Check sheet for the modelled part. Datum: model origin and axes. Units: mm. Face numbers are marked on the shaded views. Give positions to 0.01 mm unless a question says otherwise; leave off trailing zeros. Order: outer loops, then holes, each group sorted by start corner. A loop starts at its lowest first (then second) coordinate and runs counter-clockwise, first axis right, second up.
```python
from build123d import *

# Parameters (mm, degrees)
F1_DEPTH = 1.2
F2_R     = 14
F2_R_2   = 13
F3_DEPTH = 9
F5_DEPTH = 25


with BuildPart() as f1:
    # F0 (on Top) → F1 (new body)
    with BuildSketch(Plane.XY):
        with BuildLine():
            ThreePointArc((0, 55), (-38.890873, 38.890873), (-55, 0))
            ThreePointArc((-55, 0), (-38.890873, -38.890873), (0, -55))
            ThreePointArc((0, -55), (38.890873, -38.890873), (55, 0))
            ThreePointArc((55, 0), (38.890873, 38.890873), (0, 55))
        make_face()
        with BuildLine():
            ThreePointArc((-6, -41.024383), (-7.11965, -43.361964), (-9.642857, -43.954696))
            ThreePointArc((-9.642857, -43.954696), (-31.819805, -31.819805), (-43.954696, -9.642857))
            ThreePointArc((-43.954696, -9.642857), (-43.361964, -7.11965), (-41.024383, -6))
            Line((-41.024383, -6), (-15.588457, -6))
            ThreePointArc((-15.588457, -6), (-14.088457, -6.401924), (-12.990381, -7.5))
            ThreePointArc((-12.990381, -7.5), (-10.606602, -10.606602), (-7.5, -12.990381))
            ThreePointArc((-7.5, -12.990381), (-6.401924, -14.088457), (-6, -15.588457))
            Line((-6, -15.588457), (-6, -41.024383))
        make_face(mode=Mode.SUBTRACT)
        with BuildLine():
            ThreePointArc((41.024383, -6), (43.361964, -7.11965), (43.954696, -9.642857))
            ThreePointArc((43.954696, -9.642857), (31.819805, -31.819805), (9.642857, -43.954696))
            ThreePointArc((9.642857, -43.954696), (7.11965, -43.361964), (6, -41.024383))
            Line((6, -41.024383), (6, -15.588457))
            ThreePointArc((6, -15.588457), (6.401924, -14.088457), (7.5, -12.990381))
            ThreePointArc((7.5, -12.990381), (10.606602, -10.606602), (12.990381, -7.5))
            ThreePointArc((12.990381, -7.5), (14.088457, -6.401924), (15.588457, -6))
            Line((15.588457, -6), (41.024383, -6))
        make_face(mode=Mode.SUBTRACT)
        with BuildLine():
            ThreePointArc((-7.5, 12.990381), (-10.606602, 10.606602), (-12.990381, 7.5))
            ThreePointArc((-12.990381, 7.5), (-14.088457, 6.401924), (-15.588457, 6))
            Line((-15.588457, 6), (-41.024383, 6))
            ThreePointArc((-41.024383, 6), (-43.361964, 7.11965), (-43.954696, 9.642857))
            ThreePointArc((-43.954696, 9.642857), (-31.819805, 31.819805), (-9.642857, 43.954696))
            ThreePointArc((-9.642857, 43.954696), (-7.11965, 43.361964), (-6, 41.024383))
            Line((-6, 41.024383), (-6, 15.588457))
            ThreePointArc((-6, 15.588457), (-6.401924, 14.088457), (-7.5, 12.990381))
        make_face(mode=Mode.SUBTRACT)
        with BuildLine():
            ThreePointArc((6, 41.024383), (7.11965, 43.361964), (9.642857, 43.954696))
            ThreePointArc((9.642857, 43.954696), (31.819805, 31.819805), (43.954696, 9.642857))
            ThreePointArc((43.954696, 9.642857), (43.361964, 7.11965), (41.024383, 6))
            Line((41.024383, 6), (15.588457, 6))
            ThreePointArc((15.588457, 6), (14.088457, 6.401924), (12.990381, 7.5))
            ThreePointArc((12.990381, 7.5), (10.606602, 10.606602), (7.5, 12.990381))
            ThreePointArc((7.5, 12.990381), (6.401924, 14.088457), (6, 15.588457))
            Line((6, 15.588457), (6, 41.024383))
        make_face(mode=Mode.SUBTRACT)
    extrude(amount=F1_DEPTH)

    # F2 (on Top) → F3 (join)
    with BuildSketch(Plane.XY):
        Circle(F2_R)
        Circle(F2_R_2, mode=Mode.SUBTRACT)
    extrude(amount=F3_DEPTH)

    # F4 (on Top) → F5 (cut)
    with BuildSketch(Plane.XY):
        with BuildLine():
            ThreePointArc((-6.149095, -2.106806), (-5.916805, -2.690989), (-5.629165, -3.25))
            ThreePointArc((-5.629165, -3.25), (-5.288867, -3.778608), (-4.899095, -4.271869))
            ThreePointArc((-4.899095, -4.271869), (0, -6.5), (4.899095, -4.271869))
            ThreePointArc((4.899095, -4.271869), (5.288867, -3.778608), (5.629165, -3.25))
            ThreePointArc((5.629165, -3.25), (5.916805, -2.690989), (6.149095, -2.106806))
            ThreePointArc((6.149095, -2.106806), (5.629165, 3.25), (1.25, 6.378675))
            ThreePointArc((1.25, 6.378675), (0.627937, 6.469598), (0, 6.5))
            ThreePointArc((0, 6.5), (-0.627937, 6.469598), (-1.25, 6.378675))
            ThreePointArc((-1.25, 6.378675), (-5.629165, 3.25), (-6.149095, -2.106806))
        make_face()
        with BuildLine():
            ThreePointArc((-4.899095, -4.271869), (-5.288867, -3.778608), (-5.629165, -3.25))
            ThreePointArc((-5.629165, -3.25), (-5.916805, -2.690989), (-6.149095, -2.106806))
            Line((-6.149095, -2.106806), (-8.592399, -3.517448))
            ThreePointArc((-8.592399, -3.517448), (-9.211654, -4.277101), (-9.093267, -5.25))
            ThreePointArc((-9.093267, -5.25), (-8.309905, -5.838976), (-7.342399, -5.682512))
            Line((-7.342399, -5.682512), (-4.899095, -4.271869))
        make_face()
        with BuildLine():
            ThreePointArc((5.629165, -3.25), (5.288867, -3.778608), (4.899095, -4.271869))
            Line((4.899095, -4.271869), (7.342399, -5.682512))
            ThreePointArc((7.342399, -5.682512), (8.309905, -5.838976), (9.093267, -5.25))
            ThreePointArc((9.093267, -5.25), (9.211654, -4.277101), (8.592399, -3.517448))
            Line((8.592399, -3.517448), (6.149095, -2.106806))
            ThreePointArc((6.149095, -2.106806), (5.916805, -2.690989), (5.629165, -3.25))
        make_face()
        with BuildLine():
            Line((-1.25, 9.19996), (-1.25, 6.378675))
            ThreePointArc((-1.25, 6.378675), (-0.627937, 6.469598), (0, 6.5))
            ThreePointArc((0, 6.5), (0.627937, 6.469598), (1.25, 6.378675))
            Line((1.25, 6.378675), (1.25, 9.19996))
            ThreePointArc((1.25, 9.19996), (0.901749, 10.116077), (0, 10.5))
            ThreePointArc((0, 10.5), (-0.901749, 10.116077), (-1.25, 9.19996))
        make_face()
    extrude(amount=F5_DEPTH, mode=Mode.SUBTRACT)


solid = f1.part
```
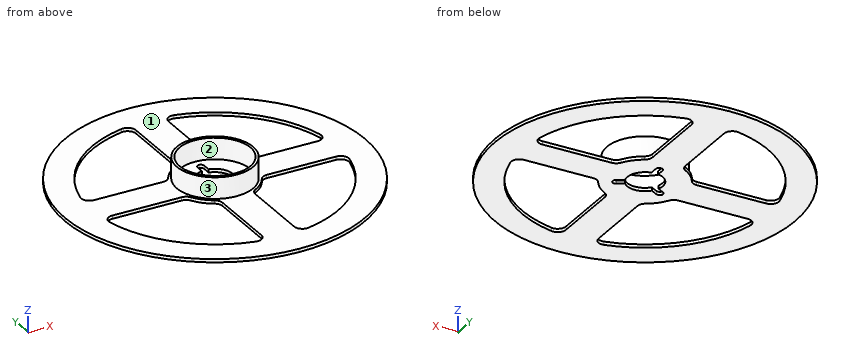
(1) Thickness scan on L1, parallel to Y at x = 0, z = 4.25; L2, parallel to X at y = -41, z = 0.5. Record the ranges inside material, lowest first.
(2) Release check for a two-part mould opening along X. For the marked faces 1, 2 and 3 record: released by +X, released by -X, zero draft, split by the parting line, or undercut.
(3) Sectioned sample at C-C (x = 3). Enter the section's corners in (y, z).
(4) Sectioned sample at B-B (y = -34). Enter the section's corners in (x, z).
(5) Go/stop test with flat-tipped pins: P1, Ø2, axis at y = -1, z = 5.5, coming from the +X side; P2, Ø1, axis at x = -40.5, y = 20, coming from the +Z side; P3, Ø0.6, axis at y = 22, z = 0.5, coming from the +X side; P4, Ø8, axis at x = -14, y = 14.5, coming from the -Z side. Record where each tip stops, or that it passes through.
(6) Sectioned sample at A-A (x = 17). Enter the section's corners in (y, z), plus the area to 3 significant figures.
(7) Sectioned sample at D-D (z = 3.25). Enter the section's corners in (x, y).
Values follow:
1. L1: y = -14 to -13, 13 to 14
1. L2: x = -36.66 to -18.55, -6 to 6, 18.55 to 36.66
2. face 1: zero draft
2. face 2: undercut
2. face 3: split by the parting line
3. outline: (-54.92, 0) - (-5.77, 0) - (-5.77, 1.2) - (-12.65, 1.2) - (-12.65, 9) - (-13.67, 9) - (-13.67, 1.2) - (-54.92, 1.2) - close; (5.77, 0) - (54.92, 0) - (54.92, 1.2) - (13.67, 1.2) - (13.67, 9) - (12.65, 9) - (12.65, 1.2) - (5.77, 1.2) - close
4. outline: (-43.23, 0) - (-29.48, 0) - (-29.48, 1.2) - (-43.23, 1.2) - close; (-6, 0) - (6, 0) - (6, 1.2) - (-6, 1.2) - close; (29.48, 0) - (43.23, 0) - (43.23, 1.2) - (29.48, 1.2) - close
5. P1: stops at x = 14
5. P2: stops at z = 1.2
5. P3: stops at x = 50.54
5. P4: passes through
6. outline: (-52.31, 0) - (-41.67, 0) - (-41.67, 1.2) - (-52.31, 1.2) - close; (-6, 0) - (6, 0) - (6, 1.2) - (-6, 1.2) - close; (41.67, 0) - (52.31, 0) - (52.31, 1.2) - (41.67, 1.2) - close
6. area: 39.9 mm2
7. outline: circle Ø28 at (0, 0); hole circle Ø26 at (0, 0)
